Can you work these out from the model? Positions are in its coordinate system, mm. Face numbers are marked on the shaded views. A direction names the side the tool comes from. Give positions to 0.01 mm unless a question says otherwise; leave off trailing zeros. Loops run counter-clockwise (first coordinate to the right, second up) from the corner with the lowest first, then second, coordinate; pieces in that order, holes last.
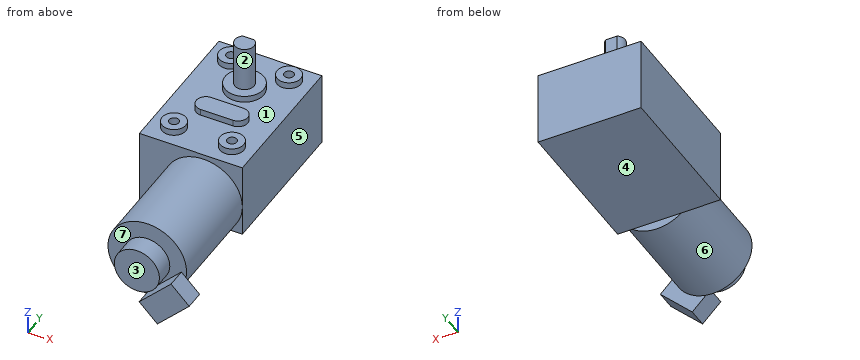
from build123d import *

# Parameters (mm, degrees)
SKETCH_372_W           = 32
SKETCH_372_H           = 46
EXTRUDE_487_DEPTH      = 23.2
SKETCH_1_R             = 12.2
EXTRUDE_677_DEPTH      = 30.8
SKETCH_726_R           = 3.7
EXTRUDE_1207_DEPTH     = 2
SKETCH_904_R           = 6
EXTRUDE_1247_DEPTH     = 2
EXTRUDE_1287_DEPTH     = 2
SKETCH_6_R             = 3
EXTRUDE_1383_DEPTH     = 14
CUT_EXTRUDE_START      = -12
CUT_EXTRUDE_1539_DEPTH = 12
SKETCH_1587_R          = 1.5
CUT_EXTRUDE_1690_DEPTH = 5
SKETCH_1732_R          = 12.2
EXTRUDE_1777_DEPTH     = 1.5
SKETCH_10_R            = 7
EXTRUDE_1879_DEPTH     = 6
EXTRUDE_2129_DEPTH     = 6


with BuildPart() as part:
    # Sketch 372 → Extrude 487 (new body)
    with BuildSketch(Plane.XY):
        with Locations((0, -8)):
            Rectangle(SKETCH_372_W, SKETCH_372_H)
    extrude(amount=EXTRUDE_487_DEPTH)

    # Эскиз1 → Extrude 677 (add)
    with BuildSketch(Plane.XZ.offset(31)):
        with Locations((3.8, 9.5)):
            Circle(SKETCH_1_R)
    extrude(amount=EXTRUDE_677_DEPTH)

    # Sketch 726 → Extrude 1207 (add)
    with BuildSketch(Plane.XY.offset(23.2)):
        with Locations((-9, 9)):
            Circle(SKETCH_726_R)
        with Locations((9, 9)):
            Circle(SKETCH_726_R)
        with Locations((9, -24)):
            Circle(SKETCH_726_R)
        with Locations((-9, -24)):
            Circle(SKETCH_726_R)
    extrude(amount=EXTRUDE_1207_DEPTH)

    # Sketch 904 → Extrude 1247 (add)
    with BuildSketch(Plane.XY.offset(23.2)):
        Circle(SKETCH_904_R)
    extrude(amount=EXTRUDE_1247_DEPTH)

    # Sketch 1024 → Extrude 1287 (add)
    with BuildSketch(Plane.XY.offset(23.2)):
        with BuildLine():
            Line((-5, -10), (5, -10))
            ThreePointArc((5, -10), (8, -13), (5, -16))
            Line((5, -16), (-5, -16))
            ThreePointArc((-5, -16), (-8, -13), (-5, -10))
        make_face()
    extrude(amount=EXTRUDE_1287_DEPTH)

    # Эскиз6 → Extrude 1383 (add)
    with BuildSketch(Plane.XY.offset(25.2)):
        Circle(SKETCH_6_R)
    extrude(amount=EXTRUDE_1383_DEPTH)

    # d-вал → Cut-Extrude 1539 (cut)
    with BuildSketch(Plane.XY.offset(39.2).offset(CUT_EXTRUDE_START)):
        with BuildLine():
            Line((-1.8, 2.4), (1.8, 2.4))
            ThreePointArc((1.8, 2.4), (0, 3), (-1.8, 2.4))
        make_face()
    extrude(amount=CUT_EXTRUDE_1539_DEPTH, mode=Mode.SUBTRACT)

    # Sketch 1587 → Cut-Extrude 1690 (cut)
    with BuildSketch(Plane.XY.offset(25.2)):
        with Locations((9, 9)):
            Circle(SKETCH_1587_R)
        with Locations((9, -24)):
            Circle(SKETCH_1587_R)
        with Locations((-9, 9)):
            Circle(SKETCH_1587_R)
        with Locations((-9, -24)):
            Circle(SKETCH_1587_R)
    extrude(amount=-CUT_EXTRUDE_1690_DEPTH, mode=Mode.SUBTRACT)

    # Sketch 1732 → Extrude 1777 (add)
    with BuildSketch(Plane.XZ.offset(61.8)):
        with Locations((3.8, 9.5)):
            Circle(SKETCH_1732_R)
    extrude(amount=EXTRUDE_1777_DEPTH)

    # Эскиз10 → Extrude 1879 (add)
    with BuildSketch(Plane.XZ.offset(63.3)):
        with Locations(Location((3.8, 9.5, 0), (0, 0, 270))):
            Circle(SKETCH_10_R)
    extrude(amount=EXTRUDE_1879_DEPTH)

    # Sketch 1921 → Extrude 2129 (add)
    with BuildSketch(Plane.XZ.offset(63.3)):
        Polygon((14.406601718, 8.792893219), (20.063455967, 3.136038969), (10.163961031, -6.763455967), (4.507106781, -1.106601718), align=None)
    extrude(amount=EXTRUDE_2129_DEPTH)


solid = part.part
(1) Suppose I cut it at D-D on z = 12. List the corners of the cut face in (x, y) for me.
Returned:
outline: (-16, -31) - (-8.14, -31) - (-8.14, -63.3) - (-2.74, -63.3) - (-2.74, -69.3) - (10.34, -69.3) - (10.34, -63.3) - (15.74, -63.3) - (15.74, -31) - (16, -31) - (16, 15) - (-16, 15) - close
(2) Which directions (+Z, -Z, +X, -X, +Y, -Y) give clear straight access to the entire face, cutting with the end or side of a thin tool? Please do the marked faces 4, 5, 6 and 7.
Returned:
face 4: -Z, +X, -X, +Y
face 5: +Z, -Z, +X, +Y
face 6: none
face 7: -Y
(3) Suppose I cut it at B-B on x = 0. List the corners of the cut face in (y, z) for me, plus the area to 3 significant figures.
Returned:
outline: (-69.3, 3.62) - (-63.3, 3.62) - (-63.3, -2.09) - (-31, -2.09) - (-31, 0) - (15, 0) - (15, 23.2) - (6, 23.2) - (6, 25.2) - (3, 25.2) - (3, 27.2) - (2.4, 27.2) - (2.4, 39.2) - (-3, 39.2) - (-3, 25.2) - (-6, 25.2) - (-6, 23.2) - (-10, 23.2) - (-10, 25.2) - (-16, 25.2) - (-16, 23.2) - (-31, 23.2) - (-31, 21.09) - (-63.3, 21.09) - (-63.3, 15.38) - (-69.3, 15.38) - close
area: 2,000 mm2
(4) Suppose I cut it at C-C on y = 9. List the corners of the cut face in (x, z) for me.
Returned:
outline: (-16, 0) - (16, 0) - (16, 23.2) - (12.7, 23.2) - (12.7, 25.2) - (10.5, 25.2) - (10.5, 20.2) - (7.5, 20.2) - (7.5, 25.2) - (5.3, 25.2) - (5.3, 23.2) - (-5.3, 23.2) - (-5.3, 25.2) - (-7.5, 25.2) - (-7.5, 20.2) - (-10.5, 20.2) - (-10.5, 25.2) - (-12.7, 25.2) - (-12.7, 23.2) - (-16, 23.2) - close
(5) Please list where these lines run through material, in increasing order: probe 1 along Y at (x, z) = (9, 22.2); probe 2 along Y at (x, z) = (9, 23.6); probe 3 along Y at (x, z) = (15.5, 15.5).
Returned:
probe 1: y = -31 to -25.5, -22.5 to 7.5, 10.5 to 15
probe 2: y = -27.7 to -25.5, -22.5 to -20.3, 5.3 to 7.5, 10.5 to 12.7
probe 3: y = -31 to 15
(6) Suppose I cut it at A-A on y = -13. List the corners of the cut face in (x, z) for me, plus the area to 3 significant figures.
Returned:
outline: (-16, 0) - (16, 0) - (16, 23.2) - (8, 23.2) - (8, 25.2) - (-8, 25.2) - (-8, 23.2) - (-16, 23.2) - close
area: 774 mm2
(7) Will these pins go through, and if not, where does the flat tip stop? P1, Ø1.8, axis at x = 9, y = 9, coming from the -Z side; P2, Ø4, axis at x = 4.5, y = -33.5, coming from the +Z side; P3, Ø3, axis at y = -24.5, z = 1, coming from the +X side.
Returned:
P1: stops at z = 0
P2: stops at z = 21.7
P3: stops at x = 16
(8) Thinking about a two-plate mould opening in Y: for the marked faces 1, 2 and 3, which applies, pulls with the +Y half, pulls with the -Y half, needs draft (parallel to the pull), parting line crosses it, or undercut?
Returned:
face 1: undercut
face 2: parting line crosses it
face 3: pulls with the -Y half
